Drawing for the job (mm, zero at the part's lowest x, y, z). Round coordinates to 2 decimals unless told otherwise and drop trailing zeros. Write each loop counter-clockwise with the first axis right and the second up, starting at its lowest first coordinate (ties: lowest second). Pieces come first, ordered by that corner, then holes.
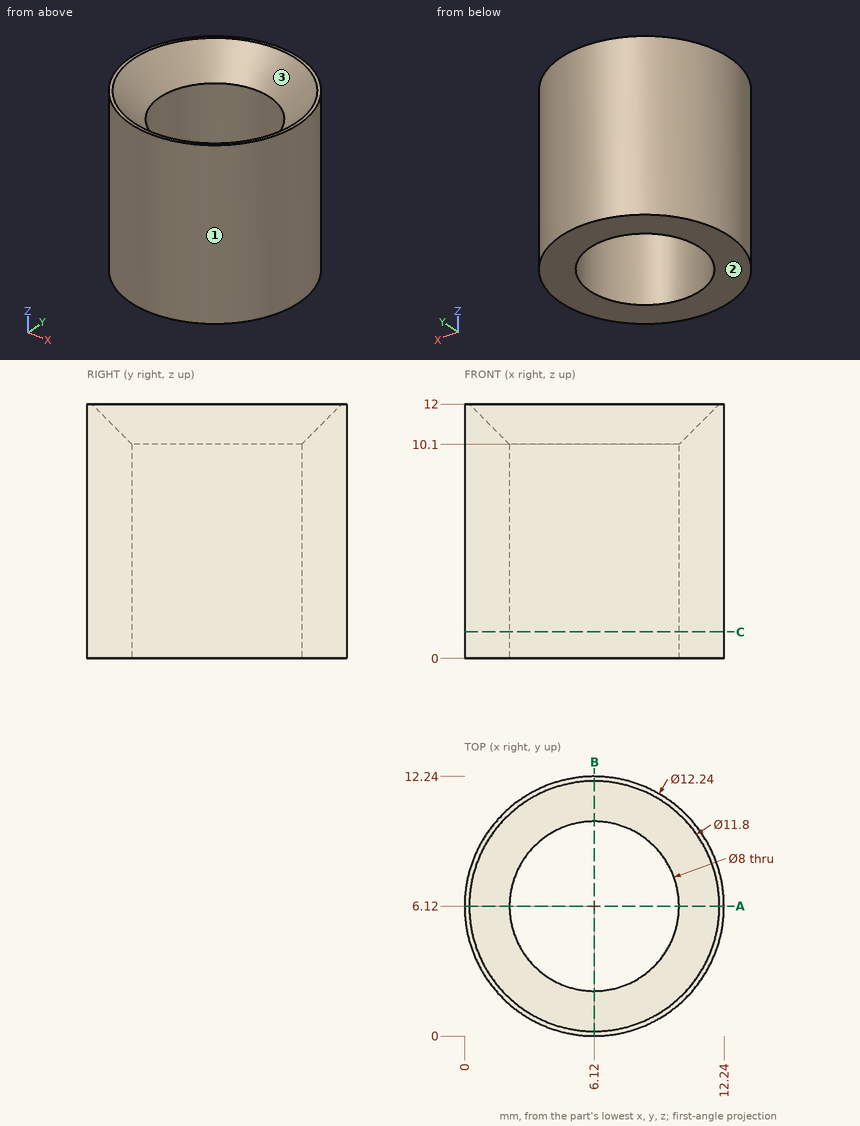
Q1. Wall check: line 1 (Y direction, x = 6.12, z = 2); line 2 (Y direction, x = 3.25, z = 6). Give the ranges that are in metal, low to high.
Q2. Saw through at A-A, the plane y = 6.12. Write the cut outline in (x, z).
Q3. Drop flat-ended pins along their axis: P1, Ø1, axis at y = 5, z = 3, coming from the +X side; P2, Ø4, axis at x = 1.5, z = 2, coming from the +Y side; P3, Ø6, axis at x = 3.5, y = 5.5, coming from the -Z side; P4, Ø5, axis at y = 10.5, z = 9, coming from the -X side. Give the stop position or say it passes through.
Q4. Two-plate mould, pull along Y, no slides. Class the marked faces 1, 2 and 3: released by +Y, released by -Y, zero draft, split by the parting line, or undercut.
Q5. Saw through at C-C, the plane z = 1.25. Write the cut outline in (x, y), and give its area (3 significant figures).
Computed:
1. line 1: y = 0 to 2.12, 10.12 to 12.24
1. line 2: y = 0.71 to 3.33, 8.91 to 11.53
2. outline: (0, 0) - (2.12, 0) - (2.12, 10.1) - (0.22, 12) - (0, 12) - close; (10.12, 0) - (12.24, 0) - (12.24, 12) - (12.02, 12) - (10.12, 10.1) - close
3. P1: stops at x = 12.21
3. P2: stops at y = 11.65
3. P3: stops at z = 0
3. P4: stops at x = 0.3
4. face 1: split by the parting line
4. face 2: zero draft
4. face 3: undercut
5. outline: circle Ø12.24 at (6.12, 6.12); hole circle Ø8 at (6.12, 6.12)
5. area: 67.4 mm2
